from build123d import *

# Parameters (mm, degrees)
SKETCH2_R                = 15.343994309
BOSS_EXTRUDE1_DEPTH      = 21
CUT_EXTRUDE1_DEPTH       = 31.19728999
FILLET1_R                = 0.5
CIRPATTERN1_COUNT        = 20
FILLET1_OF_CIRPATTERN1_R = 0.5
CUT_EXTRUDE2_DEPTH       = 31.051908029
SKETCH7_R                = 18.5
BOSS_EXTRUDE2_DEPTH      = 1


with BuildPart() as part:
    # Sketch2 → Boss-Extrude1 (new body)
    with BuildSketch(Plane.XY):
        with Locations(Location((0, 0, 0), (0, 0, 180))):
            Circle(SKETCH2_R)
    extrude(amount=BOSS_EXTRUDE1_DEPTH)

    # Sketch3 → Cut-Extrude1 (cut, through all)
    with BuildSketch(Plane(origin=(0, 0, 0), x_dir=(-1, 0, 0), z_dir=(0, 0, -1))):
        with BuildLine():
            Line((-1.614471729, 15.258821789), (-1.56, 14.743994309))
            ThreePointArc((-1.56, 14.743994309), (0, 13.183994309), (1.56, 14.743994309))
            Line((1.56, 14.743994309), (1.614471729, 15.258821789))
            ThreePointArc((1.614471729, 15.258821789), (0, 15.343994309), (-1.614471729, 15.258821789))
        make_face()
    cut_extrude1 = extrude(amount=-CUT_EXTRUDE1_DEPTH, mode=Mode.SUBTRACT)

    # Fillet1
    fillet1_edges = [part.edges().sort_by_distance(p)[0] for p in [
        (1.614471729, 15.258821789, 10.5),
        (-1.614471729, 15.258821789, 10.5),
    ]]
    fillet(fillet1_edges, radius=FILLET1_R)

    # CirPattern1: Cut-Extrude1 ×20 about axis
    cirpattern1_axis = Axis((0, 0, 0), (0, 0, 1))
    for i in range(1, CIRPATTERN1_COUNT):
        add(cut_extrude1.rotate(cirpattern1_axis, i * 360 / CIRPATTERN1_COUNT), mode=Mode.SUBTRACT)

    # Fillet1 of CirPattern1
    fillet1_of_cirpattern1_edges = [part.edges().sort_by_distance(p)[0] for p in [
        (-3.179781388, 15.010901095, 10.5),
        (-6.250689106, 14.013102692, 10.5),
        (-7.662775349, 13.293608814, 10.5),
        (-10.275045481, 11.395683469, 10.5),
        (-11.395683469, 10.275045481, 10.5),
        (-13.293608814, 7.662775349, 10.5),
        (-14.013102692, 6.250689106, 10.5),
        (-15.010901095, 3.179781388, 10.5),
        (-15.258821789, 1.614471729, 10.5),
        (-15.258821789, -1.614471729, 10.5),
        (-15.010901095, -3.179781388, 10.5),
        (-14.013102692, -6.250689106, 10.5),
        (-13.293608814, -7.662775349, 10.5),
        (-11.395683469, -10.275045481, 10.5),
        (-10.275045481, -11.395683469, 10.5),
        (-7.662775349, -13.293608814, 10.5),
        (-6.250689106, -14.013102692, 10.5),
        (-3.179781388, -15.010901095, 10.5),
        (-1.614471729, -15.258821789, 10.5),
        (1.614471729, -15.258821789, 10.5),
        (3.179781388, -15.010901095, 10.5),
        (6.250689106, -14.013102692, 10.5),
        (7.662775349, -13.293608814, 10.5),
        (10.275045481, -11.395683469, 10.5),
        (11.395683469, -10.275045481, 10.5),
        (13.293608814, -7.662775349, 10.5),
        (14.013102692, -6.250689106, 10.5),
        (15.010901095, -3.179781388, 10.5),
        (15.258821789, -1.614471729, 10.5),
        (15.258821789, 1.614471729, 10.5),
        (15.010901095, 3.179781388, 10.5),
        (14.013102692, 6.250689106, 10.5),
        (13.293608814, 7.662775349, 10.5),
        (11.395683469, 10.275045481, 10.5),
        (10.275045481, 11.395683469, 10.5),
        (7.662775349, 13.293608814, 10.5),
        (6.250689106, 14.013102692, 10.5),
        (3.179781388, 15.010901095, 10.5),
    ]]
    fillet(fillet1_of_cirpattern1_edges, radius=FILLET1_OF_CIRPATTERN1_R)

    # Sketch5 → Cut-Extrude2 (cut, through all)
    with BuildSketch(Plane(origin=(0, 0, 0), x_dir=(-1, 0, 0), z_dir=(0, 0, -1))):
        Polygon((0, -7.332348419), (6.35, -3.666174209), (6.35, 3.666174209), (0, 7.332348419), (-6.35, 3.666174209), (-6.35, -3.666174209), align=None)
    extrude(amount=-CUT_EXTRUDE2_DEPTH, mode=Mode.SUBTRACT)

    # Sketch7 → Boss-Extrude2 (add)
    with BuildSketch(Plane.XY.offset(21)):
        Circle(SKETCH7_R)
        Polygon((6.35, -3.666174209), (0, -7.332348419), (-6.35, -3.666174209), (-6.35, 3.666174209), (0, 7.332348419), (6.35, 3.666174209), align=None, mode=Mode.SUBTRACT)
    boss_extrude2 = extrude(amount=BOSS_EXTRUDE2_DEPTH)

    # Mirror1: Boss-Extrude2 across plane
    add(boss_extrude2.mirror(Plane.XY.offset(10.5)))


solid = part.part
Could you check a few things on this model? Use its own coordinates, in mm. A direction names the side the tool comes from. Coordinates: 2 decimals unless noted, no trailing zeros. Loops run counter-clockwise (first coordinate to the right, second up) from the corner with the lowest first, then second, coordinate; pieces in that order, holes last.
1. We'd pull the mould along Y, two halves only. Please class faces 5 (the face through (-12.55, -4.04, 10.35)), 6 (the face through (-4.01, -18.06, 21.49)), 7 (the face through (0.034, 13.184, 10.353)): released by +Y, released by -Y, zero draft, split by the parting line, or undercut.
2. I need wall thicknesses on L1, parallel to Z at x = -14.5, y = -4; L2, parallel to X at y = 2, z = 1.75; L3, parallel to Y at x = 13, z = 18 (3 decimals). Which ranges of each line are inside material? Lowest first, please.
3. For faces 1 (the face through (-13.184, 0.034, 10.353)), 2 (the face through (7.72, -10.69, 10.35)), 3 (the face through (8, 0, -1)), 4 (the face through (3.219, -5.474, 10.661)), which set-ups out of +Z, -Z, +X, -X, +Y, -Y let a thin tool reach every point of the face, with its end or its side?
4. Imagine slicing it at B-B (y = 0). Please give me the cut outline in (x, z), and give its area (3 significant figures).
5. Imagine slicing it at C-C (y = 5). Please give me the cut outline in (x, z).
6. Imagine slicing it at A-A (y = 16). Please give me the cut outline in (x, z), and give its area (3 significant figures).
7. For P1, Ø3, axis at y = -13.5, z = 14, coming from the -X side; P2, Ø3.5, axis at y = -1, z = 6, coming from the +X side; P3, Ø8, axis at x = -13.5, z = 9, coming from the -Y side, each with a flat end and sliding along its axis, tell me the tip position at first contact or that it passes through.
Computed values:
1. face 5: undercut
1. face 6: split by the parting line
1. face 7: released by +Y
2. L1: z = -1 to 0, 21 to 22
2. L2: x = -15.2 to -6.35, 6.35 to 15.2
2. L3: y = -7.465 to -5.734, -3.378 to 3.378, 5.734 to 7.465
3. face 1: -X
3. face 2: none
3. face 3: -Z, +X, -X, +Y, -Y
3. face 4: +Z, -Z
4. outline: (-18.5, -1) - (-6.35, -1) - (-6.35, 22) - (-18.5, 22) - (-18.5, 21) - (-13.18, 21) - (-13.18, 0) - (-18.5, 0) - close; (6.35, -1) - (18.5, -1) - (18.5, 0) - (13.18, 0) - (13.18, 21) - (18.5, 21) - (18.5, 22) - (6.35, 22) - close
4. area: 336 mm2
5. outline: (-17.81, -1) - (-4.04, -1) - (-4.04, 22) - (-17.81, 22) - (-17.81, 21) - (-12.53, 21) - (-12.53, 0) - (-17.81, 0) - close; (4.04, -1) - (17.81, -1) - (17.81, 0) - (12.53, 0) - (12.53, 21) - (17.81, 21) - (17.81, 22) - (4.04, 22) - close
6. outline: (-9.29, -1) - (9.29, -1) - (9.29, 0) - (-9.29, 0) - close; (-9.29, 21) - (9.29, 21) - (9.29, 22) - (-9.29, 22) - close
6. area: 37.1 mm2
7. P1: stops at x = -7.48
7. P2: stops at x = 15.2
7. P3: stops at y = -11.18
